```python
from build123d import *

# Parameters (mm, degrees)
F0_W         = 30
F0_H         = 14
F0_R         = 0.2
F0_W_2       = 10
F0_H_2       = 0.4
F0_R_2       = 0.3
F0_R_3       = 0.4
F0_H_3       = 0.6
F0_H_4       = 0.8
F0_H_5       = 0.3
F0_R_4       = 0.15
F0_H_6       = 0.5
F0_R_5       = 0.25
F0_R_6       = 0.5
F0_H_7       = 1
F0_R_7       = 0.6
F0_H_8       = 1.2
F0_H_9       = 0.7
F0_R_8       = 0.35
F1_DEPTH     = 6.5
F2_DEPTH     = 3.5
F3_W         = 30
F3_H         = 14
F4_DEPTH     = 1
F5_R         = 2
F6_T1_DEPTH  = 16.5
F6_T4_ANGLE  = 90
F6_T6_ANGLE  = 90
F6_T8_ANGLE  = 90
F6_T10_ANGLE = 90


# Not quite as in the source:
# - a fillet or chamfer that OpenCascade refuses, or shapes differently, is made with other operations: its cross-section is extruded or revolved along the edge and cut away or added


with BuildPart() as f1:
    # F0 (on Front) → F1 (new body)
    with BuildSketch(Plane.XZ):
        with Locations((11, -5)):
            Rectangle(F0_W, F0_H)
        with Locations((-2, -10)):
            Circle(F0_R, mode=Mode.SUBTRACT)
        with Locations((5, -9.8)):
            Rectangle(F0_W_2, F0_H_2, mode=Mode.SUBTRACT)
        with Locations((-2, -8.1)):
            Circle(F0_R_2, mode=Mode.SUBTRACT)
        with Locations((-2, -6)):
            Circle(F0_R_3, mode=Mode.SUBTRACT)
        with Locations((5, -7.8)):
            Rectangle(F0_W_2, F0_H_3, mode=Mode.SUBTRACT)
        with Locations((5, -5.6)):
            Rectangle(F0_W_2, F0_H_4, mode=Mode.SUBTRACT)
        with Locations((17, -9.75)):
            Rectangle(F0_W_2, F0_H_5, mode=Mode.SUBTRACT)
        with Locations((24, -9.9)):
            Circle(F0_R_4, mode=Mode.SUBTRACT)
        with Locations((17, -7.7)):
            Rectangle(F0_W_2, F0_H_2, mode=Mode.SUBTRACT)
        with Locations((17, -5.45)):
            Rectangle(F0_W_2, F0_H_6, mode=Mode.SUBTRACT)
        with Locations((24, -7.9)):
            Circle(F0_R, mode=Mode.SUBTRACT)
        with Locations((24, -5.7)):
            Circle(F0_R_5, mode=Mode.SUBTRACT)
        with Locations((-2, -3.7)):
            Circle(F0_R_6, mode=Mode.SUBTRACT)
        with Locations((5, -3.2)):
            Rectangle(F0_W_2, F0_H_7, mode=Mode.SUBTRACT)
        with Locations((-2, -1.2)):
            Circle(F0_R_7, mode=Mode.SUBTRACT)
        with Locations((5, -0.6)):
            Rectangle(F0_W_2, F0_H_8, mode=Mode.SUBTRACT)
        with Locations((17, -3)):
            Rectangle(F0_W_2, F0_H_3, mode=Mode.SUBTRACT)
        with Locations((24, -3.3)):
            Circle(F0_R_2, mode=Mode.SUBTRACT)
        with Locations((17, -0.35)):
            Rectangle(F0_W_2, F0_H_9, mode=Mode.SUBTRACT)
        with Locations((24, -0.7)):
            Circle(F0_R_8, mode=Mode.SUBTRACT)
        with Locations((17, -0.35)):
            Rectangle(F0_W_2, F0_H_9)
        with Locations((17, -3)):
            Rectangle(F0_W_2, F0_H_3)
        with Locations((17, -5.45)):
            Rectangle(F0_W_2, F0_H_6)
        with Locations((17, -7.7)):
            Rectangle(F0_W_2, F0_H_2)
        with Locations((17, -9.75)):
            Rectangle(F0_W_2, F0_H_5)
        with Locations((24, -0.7)):
            Circle(F0_R_8)
        with Locations((24, -3.3)):
            Circle(F0_R_2)
        with Locations((24, -5.7)):
            Circle(F0_R_5)
        with Locations((24, -7.9)):
            Circle(F0_R)
        with Locations((24, -9.9)):
            Circle(F0_R_4)
    extrude(amount=-F1_DEPTH)

    # F0 (on Front) → F2 (join)
    with BuildSketch(Plane.XZ):
        with Locations((17, -0.35)):
            Rectangle(F0_W_2, F0_H_9)
        with Locations((17, -3)):
            Rectangle(F0_W_2, F0_H_3)
        with Locations((17, -5.45)):
            Rectangle(F0_W_2, F0_H_6)
        with Locations((17, -7.7)):
            Rectangle(F0_W_2, F0_H_2)
        with Locations((17, -9.75)):
            Rectangle(F0_W_2, F0_H_5)
        with Locations((24, -0.7)):
            Circle(F0_R_8)
        with Locations((24, -3.3)):
            Circle(F0_R_2)
        with Locations((24, -5.7)):
            Circle(F0_R_5)
        with Locations((24, -7.9)):
            Circle(F0_R)
        with Locations((24, -9.9)):
            Circle(F0_R_4)
    extrude(amount=F2_DEPTH)

    # F3 (on face) → F4 (join)
    with BuildSketch(Plane(origin=(0, 6.5, 0), x_dir=(-1, 0, 0), z_dir=(0, 1, 0))):
        with Locations((-11, -5)):
            Rectangle(F3_W, F3_H)
    extrude(amount=-F4_DEPTH)

    # F5
    f5_edges = [f1.edges().sort_by_distance(p)[0] for p in [
        (-4, 6.5, -5),
        (11, 6.5, -12),
        (26, 6.5, -5),
        (11, 6.5, 2),
    ]]
    fillet(f5_edges, radius=F5_R)

    # F6: fillet of radius 4 on 4 edges, made by hand

    # F6_s2 → F6_t1 (cut)
    with BuildSketch(Plane.XZ.offset(-6.5)):
        with BuildLine():
            ThreePointArc((-4, -8), (-2.8284271247, -10.8284271247), (0, -12))
            Line((0, -12), (-4, -12))
            Line((-4, -12), (-4, -8))
        make_face()
        with BuildLine():
            ThreePointArc((0, 2), (-2.8284271247, 0.8284271247), (-4, -2))
            Line((-4, -2), (-4, 2))
            Line((-4, 2), (0, 2))
        make_face()
        with BuildLine():
            ThreePointArc((26, -8), (24.8284271247, -10.8284271247), (22, -12))
            Line((22, -12), (26, -12))
            Line((26, -12), (26, -8))
        make_face()
        with BuildLine():
            ThreePointArc((22, 2), (24.8284271247, 0.8284271247), (26, -2))
            Line((26, -2), (26, 2))
            Line((26, 2), (22, 2))
        make_face()
    extrude(amount=F6_T1_DEPTH, mode=Mode.SUBTRACT)

    # F6_s3 → F6_t4 (revolve, cut)
    with BuildSketch(Plane.YZ.offset(22)):
        with BuildLine():
            ThreePointArc((6.5, 0), (5.9142135624, 1.4142135624), (4.5, 2))
            Line((4.5, 2), (6.5, 2))
            Line((6.5, 2), (6.5, 0))
        make_face()
    revolve(axis=Axis((22, 6.5, -2), (0, 1, 0)), revolution_arc=F6_T4_ANGLE, mode=Mode.SUBTRACT)

    # F6_s5 → F6_t6 (revolve, cut)
    with BuildSketch(Plane.XY.offset(-8)):
        with BuildLine():
            ThreePointArc((24, 6.5), (25.4142135624, 5.9142135624), (26, 4.5))
            Line((26, 4.5), (26, 6.5))
            Line((26, 6.5), (24, 6.5))
        make_face()
    revolve(axis=Axis((22, 6.5, -8), (0, 1, 0)), revolution_arc=F6_T6_ANGLE, mode=Mode.SUBTRACT)

    # F6_s7 → F6_t8 (revolve, cut)
    with BuildSketch(Plane.XY.offset(-2)):
        with BuildLine():
            ThreePointArc((-2, 6.5), (-3.4142135624, 5.9142135624), (-4, 4.5))
            Line((-4, 4.5), (-4, 6.5))
            Line((-4, 6.5), (-2, 6.5))
        make_face()
    revolve(axis=Axis((0, 6.5, -2), (0, 1, 0)), revolution_arc=F6_T8_ANGLE, mode=Mode.SUBTRACT)

    # F6_s9 → F6_t10 (revolve, cut)
    with BuildSketch(Plane.YZ):
        with BuildLine():
            ThreePointArc((6.5, -10), (5.9142135624, -11.4142135624), (4.5, -12))
            Line((4.5, -12), (6.5, -12))
            Line((6.5, -12), (6.5, -10))
        make_face()
    revolve(axis=Axis((0, 6.5, -8), (0, 1, 0)), revolution_arc=F6_T10_ANGLE, mode=Mode.SUBTRACT)


solid = f1.part
```
Model file for the job. Use its own axes, mm. A direction names the side the tool comes from. Give positions to 0.01 mm unless a question says otherwise; leave off trailing zeros. Write each loop counter-clockwise with the first axis right and the second up, starting at its lowest first coordinate (ties: lowest second). Pieces come first, ordered by that corner, then holes. Notation, with made-up numbers: (85.25, -12) - (103.25, -12) arc R18 ccw to (103.25, -7) - close; hole circle Ø11 at (40.5, -26.75). An arc over 180 degrees is marked (long way). One line per question, with ' | ' between items. Start each with the question number.
(1) Pin check, flat tips, straight feed: P1, Ø1, axis at x = 17, y = -2.5, coming from the +Z side; P2, Ø1.3, axis at x = -2, z = -1, coming from the -Y side; P3, Ø1.8, axis at x = 18.5, y = -1, coming from the -Z side. Stop position of each tip, or through.
(2) 3-axis set-ups, long thin cutter, end or side, ignore diameter. For faces 5 (the face through (5, 5.5, -3)), 6 (the face through (17, -2, -5.7)), 7 (the face through (17, -2, -9.9)), 8 (the face through (17, -2, 0)), 9 (the face through (11, 2, 2)): which of +Z, -Z, +X, -X, +Y, -Y reach the whole face in a straight line?
(3) Slice it at A-A on y = -1.75. Give the number of separate pieces and of enclosed holes in the cut face, plus the area to 3 significant figures.
(4) Wall check: line 1 along Z through (x, y) = (4, 2); line 2 along Z through (x, y) = (-2, 1.7); line 3 along X through (y, z) = (4.75, -1.5). Give the ranges that are in metal, low to high. Write a range as from..to.
(5) Slice it at D-D on x = 19. Write the cut outline in (y, z), plus the area to 3 significant figures.
(6) Slice it at C-C on x = 7. Write the cut outline in (y, z), plus the area to 3 significant figures.
(7) Two-plate mould, pull along X, no slides. Class faces 1 (the face through (26, 2, -5)), 2 (the face through (17, -2, -0.7)), 3 (the face through (0, 3, -1)), 4 (the face through (5, 3, -3.7)): +X half, -X half, draft (parallel to the pull), parting line (faces both ways), or undercut.
Results below:
1) P1: z = 0 | P2: y = 0 | P3: z = -9.9
2) face 5: -Y | face 6: -X, -Y | face 7: -Z, -X, -Y | face 8: +Z, +X, -X, -Y | face 9: +Z, +X, -X, +Y, -Y
3) separate pieces: 10 | enclosed holes: 0 | area: 26.1 mm^2
4) line 1: -12..-10, -9.6..-8.1, -7.5..-6, -5.2..-3.7, -2.7..-1.2, 0..2 | line 2: -11.46..-10.2, -9.8..-8.4, -7.8..-6.4, -5.6..-4.2, -3.2..-1.8, -0.6..1.46 | line 3: -3.95..-2.52, -1.48..25.95
5) outline: (-3.5, -9.9) - (0, -9.9) - (0, -12) - (4.5, -12) arc R2 ccw to (6.5, -10) - (6.5, 0) arc R2 ccw to (4.5, 2) - (0, 2) - (0, 0) - (-3.5, 0) - (-3.5, -0.7) - (0, -0.7) - (0, -2.7) - (-3.5, -2.7) - (-3.5, -3.3) - (0, -3.3) - (0, -5.2) - (-3.5, -5.2) - (-3.5, -5.7) - (0, -5.7) - (0, -7.5) - (-3.5, -7.5) - (-3.5, -7.9) - (0, -7.9) - (0, -9.6) - (-3.5, -9.6) - close | area: 98.0 mm^2
6) outline: (0, -12) - (4.5, -12) arc R2 ccw to (6.5, -10) - (6.5, 0) arc R2 ccw to (4.5, 2) - (0, 2) - (0, 0) - (5.5, 0) - (5.5, -1.2) - (0, -1.2) - (0, -2.7) - (5.5, -2.7) - (5.5, -3.7) - (0, -3.7) - (0, -5.2) - (5.5, -5.2) - (5.5, -6) - (0, -6) - (0, -7.5) - (5.5, -7.5) - (5.5, -8.1) - (0, -8.1) - (0, -9.6) - (5.5, -9.6) - (5.5, -10) - (0, -10) - close | area: 67.3 mm^2
7) face 1: +X half | face 2: draft | face 3: undercut | face 4: undercut
